Part model, mm, in its own coordinate system. A direction names the side the tool comes from. Round coordinates to 2 decimals unless told otherwise and drop trailing zeros. Loops run counter-clockwise (first coordinate to the right, second up) from the corner with the lowest first, then second, coordinate; pieces in that order, holes last. Notation, with made-up numbers: (-8, 33) -> (49, 33) arc R19 ccw to (49, 44) -> close; hole circle Ø5 at (-24.75, 42.25). An arc over 180 degrees is marked (long way). Answer as CSV lines item,"result".
from build123d import *

# Parameters (mm, degrees)
BOSS_EXTRUDE1_DEPTH = 47.9
SKETCH4_W           = 91.495453484
SKETCH4_H           = 57.017695921
CUT_EXTRUDE3_DEPTH  = 20
BOSS_EXTRUDE2_DEPTH = 3
FILLET1_R           = 0.5
SKETCH7_W           = 5
SKETCH7_H           = 47.9
CUT_EXTRUDE4_DEPTH  = 31
SKETCH8_W           = 14.75
SKETCH8_H           = 46.9
SKETCH8_W_2         = 14.5
CUT_EXTRUDE6_DEPTH  = 90.636878571
SKETCH9_W           = 45.35
SKETCH9_H           = 26.396021741
CUT_EXTRUDE7_DEPTH  = 3
BOSS_EXTRUDE3_DEPTH = 3
SKETCH12_W          = 22.7
SKETCH12_H          = 12.2
CUT_EXTRUDE8_DEPTH  = 104.043728582
SKETCH13_W          = 45.35
SKETCH13_H          = 5
BOSS_EXTRUDE4_DEPTH = 3
SKETCH16_R          = 2
CUT_EXTRUDE9_DEPTH  = 10
SKETCH18_R          = 2
CUT_EXTRUDE10_DEPTH = 10


with BuildPart() as part:
    # Sketch1 → Boss-Extrude1 (new body)
    with BuildSketch(Plane.XY):
        Polygon((0, 0), (0, 56), (75.6, 56), (75.6, 0), (70.6, 0), (70.6, 51), (5, 51), (5, 0), align=None)
    extrude(amount=BOSS_EXTRUDE1_DEPTH)

    # Sketch4 → Cut-Extrude3 (cut)
    with BuildSketch(Plane.XZ):
        with Locations((38.801775038, 24.20044376)):
            Rectangle(SKETCH4_W, SKETCH4_H)
    extrude(amount=-CUT_EXTRUDE3_DEPTH, mode=Mode.SUBTRACT)

    # Sketch6 → Boss-Extrude2 (add)
    with BuildSketch(Plane(origin=(0, 56, 0), x_dir=(1, 0, 0), z_dir=(0, 1, 0))):
        Polygon((26.9, -4.3), (26.9, 0), (24.9, 0), (24.9, -2.3), (20.1, -2.3), (20.1, -8.8), (24.9, -8.8), (24.9, -24.5), (51.4, -24.5), (51.4, -8.8), (56.2, -8.8), (56.2, -2.3), (51.4, -2.3), (51.4, 0), (49.4, 0), (49.4, -4.3), (54.2, -4.3), (54.2, -6.8), (49.4, -6.8), (49.4, -22.5), (26.9, -22.5), (26.9, -6.8), (22.1, -6.8), (22.1, -4.3), align=None)
    extrude(amount=BOSS_EXTRUDE2_DEPTH)

    # Fillet1
    fillet1_edges = [part.edges().sort_by_distance(p)[0] for p in [
        (0, 56, 23.95),
        (75.6, 56, 23.95),
        (37.8, 56, 47.9),
        (12.45, 56, 0),
        (24.9, 57.5, 0),
        (51.4, 57.5, 0),
        (24.9, 56, 1.15),
        (51.4, 56, 1.15),
        (53.8, 56, 2.3),
        (56.2, 56, 5.55),
        (53.8, 56, 8.8),
        (51.4, 56, 16.65),
        (38.15, 56, 24.5),
        (24.9, 56, 16.65),
        (22.5, 56, 8.8),
        (20.1, 56, 5.55),
        (22.5, 56, 2.3),
        (63.5, 56, 0),
    ]]
    fillet(fillet1_edges, radius=FILLET1_R)

    # Sketch7 → Cut-Extrude4 (cut)
    with BuildSketch(Plane.XZ.offset(-20)):
        with Locations((2.5, 23.95)):
            Rectangle(SKETCH7_W, SKETCH7_H)
        with Locations((73.1, 23.95)):
            Rectangle(SKETCH7_W, SKETCH7_H)
    extrude(amount=-CUT_EXTRUDE4_DEPTH, mode=Mode.SUBTRACT)

    # Sketch8 → Cut-Extrude6 (cut, through all)
    with BuildSketch(Plane(origin=(0, 56, 0), x_dir=(1, 0, 0), z_dir=(0, 1, 0))):
        with Locations((7.875, -23.95)):
            Rectangle(SKETCH8_W, SKETCH8_H)
        Polygon((0.25, -47.65), (0.25, 0), (0, 0), (0, -47.9), (15.25, -47.9), (15.25, -47.65), align=None)
        Polygon((15.25, -0.5), (15.25, 0), (0.25, 0), (0.25, -47.65), (15.25, -47.65), (15.25, -47.4), (0.5, -47.4), (0.5, -0.5), align=None)
        with Locations((67.85, -23.95)):
            Rectangle(SKETCH8_W_2, SKETCH8_H)
        Polygon((75.1, -47.4), (60.6, -47.4), (60.6, -47.9), (75.6, -47.9), (75.6, 0), (60.6, 0), (60.6, -0.5), (75.1, -0.5), align=None)
    extrude(amount=-CUT_EXTRUDE6_DEPTH, mode=Mode.SUBTRACT)

    # Sketch9 → Cut-Extrude7 (cut)
    with BuildSketch(Plane(origin=(0, 59, 0), x_dir=(1, 0, 0), z_dir=(0, 1, 0))):
        with Locations((37.925, -13.198010871)):
            Rectangle(SKETCH9_W, SKETCH9_H)
    extrude(amount=-CUT_EXTRUDE7_DEPTH, mode=Mode.SUBTRACT)

    # Sketch11 → Boss-Extrude3 (add)
    with BuildSketch(Plane(origin=(0, 0, 0), x_dir=(-1, 0, 0), z_dir=(0, 0, -1))):
        with BuildLine():
            Line((-50.95, 62.1), (-38.15, 62.1))
            Line((-38.15, 62.1), (-38.15, 68.2))
            Line((-38.15, 68.2), (-54.2, 68.2))
            Line((-54.2, 68.2), (-54.2, 62.1))
            Line((-54.2, 62.1), (-53.15, 62.1))
            ThreePointArc((-53.15, 62.1), (-52.05, 63.2), (-50.95, 62.1))
        make_face()
        with BuildLine():
            Line((-51.033974596, 56), (-38.15, 56))
            Line((-38.15, 56), (-38.15, 62.1))
            Line((-38.15, 62.1), (-50.95, 62.1))
            ThreePointArc((-50.95, 62.1), (-52.05, 61), (-53.15, 62.1))
            Line((-53.15, 62.1), (-54.2, 62.1))
            Line((-54.2, 62.1), (-54.2, 56))
            Line((-54.2, 56), (-51.033974596, 56))
        make_face()
        with BuildLine():
            Line((-38.15, 68.2), (-38.15, 62.1))
            Line((-38.15, 62.1), (-25.35, 62.1))
            ThreePointArc((-25.35, 62.1), (-24.25, 63.2), (-23.15, 62.1))
            Line((-23.15, 62.1), (-22.1, 62.1))
            Line((-22.1, 62.1), (-22.1, 68.2))
            Line((-22.1, 68.2), (-38.15, 68.2))
        make_face()
        with BuildLine():
            Line((-38.15, 62.1), (-38.15, 56))
            Line((-38.15, 56), (-25.266025404, 56))
            Line((-25.266025404, 56), (-22.1, 56))
            Line((-22.1, 56), (-22.1, 62.1))
            Line((-22.1, 62.1), (-23.15, 62.1))
            ThreePointArc((-23.15, 62.1), (-24.25, 61), (-25.35, 62.1))
            Line((-25.35, 62.1), (-38.15, 62.1))
        make_face()
    extrude(amount=-BOSS_EXTRUDE3_DEPTH)

    # Sketch12 → Cut-Extrude8 (cut, through all)
    with BuildSketch(Plane(origin=(0, 0, 0), x_dir=(-1, 0, 0), z_dir=(0, 0, -1))):
        with Locations((-38.15, 62.1)):
            Rectangle(SKETCH12_W, SKETCH12_H)
    extrude(amount=-CUT_EXTRUDE8_DEPTH, mode=Mode.SUBTRACT)

    # Sketch13 → Boss-Extrude4 (add)
    with BuildSketch(Plane(origin=(0, 0, 0), x_dir=(-1, 0, 0), z_dir=(0, 0, -1))):
        with Locations((-37.925, 53.5)):
            Rectangle(SKETCH13_W, SKETCH13_H)
    extrude(amount=-BOSS_EXTRUDE4_DEPTH)

    # Sketch16 → Cut-Extrude9 (cut)
    with BuildSketch(Plane(origin=(0, 56, 0), x_dir=(1, 0, 0), z_dir=(0, 1, 0))):
        with Locations(Location((33.925, -33.404714852, 0), (0, 0, 270))):
            Circle(SKETCH16_R)
        with Locations(Location((41.925, -33.404714852, 0), (0, 0, 270))):
            Circle(SKETCH16_R)
        with Locations(Location((41.925, -44.404714852, 0), (0, 0, 270))):
            Circle(SKETCH16_R)
        with Locations(Location((33.925, -44.404714852, 0), (0, 0, 270))):
            Circle(SKETCH16_R)
    extrude(amount=-CUT_EXTRUDE9_DEPTH, mode=Mode.SUBTRACT)

    # Sketch18 → Cut-Extrude10 (cut)
    with BuildSketch(Plane(origin=(0, 56, 0), x_dir=(1, 0, 0), z_dir=(0, 1, 0))):
        with Locations(Location((18.25, -12, 0), (0, 0, 270))):
            Circle(SKETCH18_R)
        with Locations(Location((57.6, -12, 0), (0, 0, 270))):
            Circle(SKETCH18_R)
    extrude(amount=-CUT_EXTRUDE10_DEPTH, mode=Mode.SUBTRACT)


solid = part.part
Q1. Drill centre lines: line 1 along X through (y, z) = (62.1, 1.5); line 2 along X through (y, z) = (53.7, 12); line 3 along Y through (x, z) = (33, 9). Where is each one in solid material? Low to high.
Geometry results:
line 1,"22.1 to 23.15, 25.35 to 26.8, 49.5 to 50.95, 53.15 to 54.2"
line 2,"15.25 to 16.25, 20.25 to 55.6, 59.6 to 60.6"
line 3,"51 to 56"
Q2. Saw through at B-B, the plane z = 12. Write the cut outline in (x, y), then the cut area to 3 significant figures.
Geometry results:
outline,"(15.25, 51) -> (16.25, 51) -> (16.25, 56) -> (15.25, 56) -> close; (20.25, 51) -> (55.6, 51) -> (55.6, 56) -> (20.25, 56) -> close; (59.6, 51) -> (60.6, 51) -> (60.6, 56) -> (59.6, 56) -> close"
area,"187 mm2"
Q3. Saw through at C-C, the plane x = 57.6. Write the cut outline in (y, z), then the cut area to 3 significant figures.
Geometry results:
outline,"(51, 0) -> (56, 0) -> (56, 10) -> (51, 10) -> close; (51, 14) -> (56, 14) -> (56, 47.4) arc R0.5 ccw to (55.5, 47.9) -> (51, 47.9) -> close"
area,"219 mm2"
Q4. Two-plate mould, pull along X, no slides. Class faces 4 (the face through (52.9, 62.8, 1.5)), 5 (the face through (52, 68.2, 1)), 6 (the face through (60.6, 54, 24)): pulls with the +X half, pulls with the -X half, needs draft (parallel to the pull), parting line crosses it, or undercut.
Geometry results:
face 4,"undercut"
face 5,"needs draft"
face 6,"pulls with the +X half"
Q5. Which spindle directions (+Z, -Z, +X, -X, +Y, -Y) get a long thin tool onto all of the face, cutting with end or side? Do faces 1 (the face through (22.1, 62, 1)), 2 (the face through (50.8, 62.2, 3)), 3 (the face through (26.8, 62, 1)). Say none if no direction does.
Geometry results:
face 1,"+Z, -Z, -X, +Y"
face 2,"+Z, +X, -X, +Y"
face 3,"+Z, -Z, +Y"
Q6. Saw through at D-D, the plane y = 62.1. Write the cut outline in (x, z).
Geometry results:
outline,"(22.1, 0) -> (23.15, 0) -> (23.15, 3) -> (22.1, 3) -> close; (25.35, 0) -> (26.8, 0) -> (26.8, 3) -> (25.35, 3) -> close; (49.5, 0) -> (50.95, 0) -> (50.95, 3) -> (49.5, 3) -> close; (53.15, 0) -> (54.2, 0) -> (54.2, 3) -> (53.15, 3) -> close"
Q7. Saw through at A-A, the plane y = 58.25. Write the cut outline in (x, z).
Geometry results:
outline,"(22.1, 0) -> (26.8, 0) -> (26.8, 3) -> (22.1, 3) -> close; (49.5, 0) -> (54.2, 0) -> (54.2, 3) -> (49.5, 3) -> close"
Q8. Drop flat-ended pins along their axis: P1, Ø6.5, axis at x = 41.92, z = 33.4, coming from the +Y side; P2, Ø4, axis at x = 52, y = 60.5, coming from the +Z side; P3, Ø1.5, axis at y = 63, z = 2, coming from the +X side. Give the stop position or say it passes through.
Geometry results:
P1,"y = 56"
P2,"z = 3"
P3,"x = 54.2"
